```python
from build123d import *

# Parameters (mm, degrees)
EXTRUDE_1_DEPTH     = 6
CUT_EXTRUDE_1_DEPTH = 2.1
CUT_EXTRUDE_2_DEPTH = 2.1


with BuildPart() as part:
    # Эскиз2 → Бобышка-Вытянуть1 (new body)
    with BuildSketch(Plane(origin=(0, 0, 0), x_dir=(1, 0, 0), z_dir=(0, 1, 0))):
        with BuildLine():
            Line((-5.696343687, 30.010357476), (-5.499915116, -19.989642524))
            ThreePointArc((-5.499915116, -19.989642524), (0.021649418, -25.467993105), (5.5, -19.946428571))
            Line((5.5, -19.946428571), (5.303571429, 30.053571429))
            ThreePointArc((5.303571429, 30.053571429), (-0.217993105, 35.53192201), (-5.696343687, 30.010357476))
        make_face()
    extrude(amount=EXTRUDE_1_DEPTH)

    # Эскиз3 → Вырез-Вытянуть1 (cut)
    with BuildSketch(Plane(origin=(0, 6, 0), x_dir=(1, 0, 0), z_dir=(0, 1, 0))):
        with BuildLine():
            Line((-3.882448388, 29.711113982), (-2.525666878, 14.123849568))
            ThreePointArc((-2.525666878, 14.123849568), (-0.125279076, 11.931987312), (2.257813124, 14.142641811))
            Line((2.257813124, 14.142641811), (3.492083281, 29.740085357))
            ThreePointArc((3.492083281, 29.740085357), (-0.210921731, 33.7319359), (-3.882448388, 29.711113982))
        make_face()
    extrude(amount=-CUT_EXTRUDE_1_DEPTH, mode=Mode.SUBTRACT)

    # Эскиз4 → Вырез-Вытянуть2 (cut)
    with BuildSketch(Plane(origin=(0, 3.9, 0), x_dir=(1, 0, 0), z_dir=(0, 1, 0))):
        with BuildLine():
            Line((-3.405520008, 24.231964452), (3.056209977, 24.231964452))
            Line((3.056209977, 24.231964452), (3.492083281, 29.740085357))
            ThreePointArc((3.492083281, 29.740085357), (-0.210921731, 33.7319359), (-3.882448388, 29.711113982))
            Line((-3.882448388, 29.711113982), (-3.405520008, 24.231964452))
        make_face()
    extrude(amount=-CUT_EXTRUDE_2_DEPTH, mode=Mode.SUBTRACT)


solid = part.part
```
Input: part model. Units: mm. Frame: model coordinates. A direction names the side the tool comes from. Give positions to 0.01 mm unless a question says otherwise; leave off trailing zeros. Order: outer loops, then holes, each group sorted by start corner. A loop starts at its lowest first (then second) coordinate and runs counter-clockwise, first axis right, second up. Notation, with made-up numbers: (55.5, -13.75) - (95.5, -13.75) arc R8 cw to (95.5, 1.25) - close; hole circle Ø5 at (47.25, 36). An arc over 180 degrees is marked (long way). Use a Markdown table: item, result.
(1) Draft query along Z for faces 3 (the flat face through (0, 3.9, -18)), 4 (the flat face through (0, 6, 1)). Return one class per face: released by +Z, released by -Z, zero draft, split by the parting line, or undercut.
Computed values:
| item | result |
|---|---|
| face 3 | undercut |
| face 4 | zero draft |
(2) Section query D-D (z = -13). Output: boundary loops of the cut face in (x, y), then the cut area to 3 significant figures.
Computed values:
| item | result |
|---|---|
| outline | (-5.63, 0) - (5.37, 0) - (5.37, 6) - (1.86, 6) - (1.86, 3.9) - (-2.13, 3.9) - (-2.13, 6) - (-5.63, 6) - close |
| area | 57.6 mm2 |
(3) Access query for faces 1 (the flat face through (0, 0, -5)), 2 (the flat face through (0, 3, -24.232)). Directions: +Z, -Z, +X, -X, +Y, -Y. A direction counts if a zero-diameter tool reaches every point of the face in a straight line with its end or side. Return the directions, or none.
Computed values:
| item | result |
|---|---|
| face 1 | +Z, -Z, +X, -X, -Y |
| face 2 | +Y |
(4) Line query: line 1 (Z direction, x = 1.5, y = 1.85); line 2 (Y direction, x = 0, z = -24); line 3 (Z direction, x = 2.5, y = 2.6). Output: solid intervals per line, ascending. Write a range as from..to.
Computed values:
| item | result |
|---|---|
| line 1 | z = -35.26..-33.32, -24.23..25.26 |
| line 2 | y = 0..3.9 |
| line 3 | z = -34.83..-32.57, -24.23..24.87 |
(5) Pin query (flat end, axial travel): pin 1 (1.5 mm diameter, centred on y = 5.5, z = 2, fed in from -X); pin 2 (0.6 mm diameter, centred on x = 1, y = 3, fed in from -Z); pin 3 (1.5 mm diameter, centred on y = 5, z = -18, fed in from -X). Return the tip coordinate at first contact, or that it passes through.
Computed values:
| item | result |
|---|---|
| pin 1 | stops at x = -5.57 |
| pin 2 | stops at z = -35.46 |
| pin 3 | stops at x = -5.65 |
(6) Section query A-A (y = 4.65). Output: boundary loops of the cut face in (x, z), then the cut area to 3 significant figures.
Computed values:
| item | result |
|---|---|
| outline | (-5.7, -30.01) arc R5.5 ccw to (5.3, -30.05) - (5.5, 19.95) arc R5.5 ccw to (-5.5, 19.99) - close; hole (-3.88, -29.71) arc R3.7 ccw (long way) to (3.49, -29.74) - (2.26, -14.14) arc R2.4 ccw to (-2.53, -14.12) - close |
| area | 518 mm2 |
(7) Section query B-B (x = -0.75). Output: boundary loops of the cut face in (y, z).
Computed values:
| item | result |
|---|---|
| outline | (0, -35.5) - (6, -35.5) - (6, -33.69) - (1.8, -33.69) - (1.8, -24.23) - (3.9, -24.23) - (3.9, -12.01) - (6, -12.01) - (6, 25.42) - (0, 25.42) - close |
(8) Section query C-C (y = 0.6). Output: boundary loops of the cut face in (x, z).
Computed values:
| item | result |
|---|---|
| outline | (-5.7, -30.01) arc R5.5 ccw to (5.3, -30.05) - (5.5, 19.95) arc R5.5 ccw to (-5.5, 19.99) - close |
